Geometry check sheet. Reference: the model listing, model coordinates, mm. Round coordinates to 2 decimals unless told otherwise and drop trailing zeros. Write each loop counter-clockwise with the first axis right and the second up, starting at its lowest first coordinate (ties: lowest second). Pieces come first, ordered by that corner, then holes.
Item 1: Scan lines: probe 1 along Y at (x, z) = (71, 1.25); probe 2 along Y at (x, z) = (0, 5.25); probe 3 along X at (y, z) = (28.5, 5.5). Record each from-to range of solid material in increasing order.
Item 2: Cross-section at A-A (z = 1.75). Enter the section's corners in (x, y).
Item 3: Cross-section at B-B (y = 20). Enter the section's corners in (x, z), then the cut area to 3 significant figures.
Item 4: Depth check by flat-ended pin: P1, Ø20, axis at x = 0, y = 20, coming from the +Z side; P2, Ø4, axis at y = 21, z = 5, coming from the +X side. Enter the tip coordinate at first touch or a pass-through.
Item 5: Cross-section at C-C (y = 34.5). Enter the section's corners in (x, z).
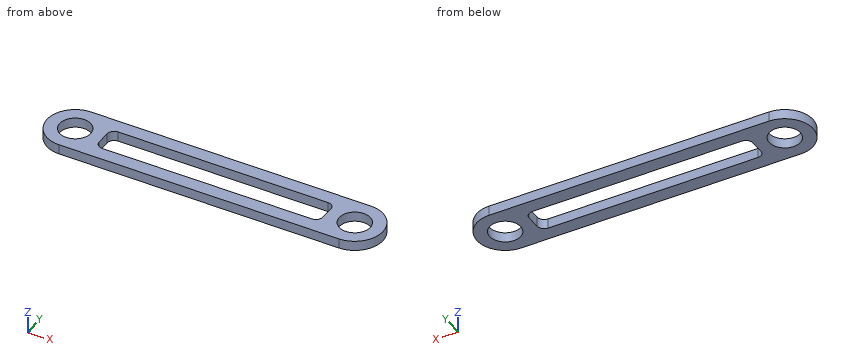
from build123d import *

# Parameters (mm, degrees)
F1_DEPTH = 7
F2_R     = 11
F2_R_2   = 10
F3_DEPTH = 7
F4_W     = 160
F4_H     = 20
F5_DEPTH = 7.001
F6_R     = 5


with BuildPart() as f1:
    # F0 (on Top) → F1 (new body)
    with BuildSketch(Plane.XY):
        with BuildLine():
            Line((0, 10), (0, 0))
            Line((0, 0), (200, 0))
            Line((200, 0), (200, 10))
            ThreePointArc((200, 10), (190, 20), (200, 30))
            Line((200, 30), (200, 40))
            Line((200, 40), (0, 40))
            Line((0, 40), (0, 30))
            ThreePointArc((0, 30), (7.071068, 27.071068), (10, 20))
            ThreePointArc((10, 20), (7.071068, 12.928932), (0, 10))
        make_face()
        with BuildLine():
            ThreePointArc((0, 40), (-20, 20), (0, 0))
            Line((0, 0), (0, 10))
            ThreePointArc((0, 10), (-10, 20), (0, 30))
            Line((0, 30), (0, 40))
        make_face()
        with BuildLine():
            Line((200, 10), (200, 0))
            ThreePointArc((200, 0), (220, 20), (200, 40))
            Line((200, 40), (200, 30))
            ThreePointArc((200, 30), (207.071068, 27.071068), (210, 20))
            ThreePointArc((210, 20), (207.071068, 12.928932), (200, 10))
        make_face()
    extrude(amount=F1_DEPTH)

    # F2 (on face) → F3 (cut)
    with BuildSketch(Plane.XY.offset(7)):
        with Locations((0, 20)):
            Circle(F2_R)
        with Locations((0, 20)):
            Circle(F2_R_2, mode=Mode.SUBTRACT)
        with Locations((200, 20)):
            Circle(F2_R)
        with Locations((200, 20)):
            Circle(F2_R_2, mode=Mode.SUBTRACT)
    extrude(amount=-F3_DEPTH, mode=Mode.SUBTRACT)

    # F4 (on face) → F5 (cut, through all)
    with BuildSketch(Plane.XY.offset(7)):
        with Locations((100, 20)):
            Rectangle(F4_W, F4_H)
    extrude(amount=-F5_DEPTH, mode=Mode.SUBTRACT)

    # F6
    f6_edges = [f1.edges().sort_by_distance(p)[0] for p in [
        (20, 30, 3.5),
        (180, 30, 3.5),
        (180, 10, 3.5),
        (20, 10, 3.5),
    ]]
    fillet(f6_edges, radius=F6_R)


solid = f1.part
Resolved:
1. probe 1: y = 0 to 10, 30 to 40
1. probe 2: y = 0 to 9, 31 to 40
1. probe 3: x = -18.1 to -6.98, 6.98 to 21.43, 178.57 to 193.02, 206.98 to 218.1
2. outline: (0, 0) - (200, 0) arc R20 ccw to (200, 40) - (0, 40) arc R20 ccw to start; hole circle Ø22 at (0, 20); hole (20, 15) arc R5 ccw to (25, 10) - (175, 10) arc R5 ccw to (180, 15) - (180, 25) arc R5 ccw to (175, 30) - (25, 30) arc R5 ccw to (20, 25) - close; hole circle Ø22 at (200, 20)
3. outline: (-20, 0) - (-11, 0) - (-11, 7) - (-20, 7) - close; (11, 0) - (20, 0) - (20, 7) - (11, 7) - close; (180, 0) - (189, 0) - (189, 7) - (180, 7) - close; (211, 0) - (220, 0) - (220, 7) - (211, 7) - close
3. area: 252 mm2
4. P1: passes through
4. P2: stops at x = 220
5. outline: (-13.77, 0) - (213.77, 0) - (213.77, 7) - (-13.77, 7) - close
